Input: part model. Units: mm. Frame: model coordinates. A direction names the side the tool comes from. Round coordinates to 2 decimals unless told otherwise and drop trailing zeros. Order: outer loops, then holes, each group sorted by start corner. A loop starts at its lowest first (then second) coordinate and runs counter-clockwise, first axis right, second up.
Item 1: Mould query, pull axis Y, two halves, no side actions, for faces 1 (the cylindrical face through (8.4, 22.8, -1)), 2 (the flat face through (1, -26, -9)), 3 (the flat face through (10, 21.7, -1)), 4 (the flat face through (-15.5, 8, -6)). Classes: released by +Y, released by -Y, zero draft, split by the parting line, or undercut.
Item 2: First-contact query: pin 1 (2 mm diameter, centred on x = 2.5, z = -7.5, fed in from +Y); pin 2 (0.7 mm diameter, centred on x = -10, y = 22.5, fed in from +Z). Flat tips, straight axial feed; report the tip coordinate or a pass-through.
Item 3: Cut plane C-C on z = -10.5. Output: boundary loops of the cut face in (x, y), then the cut area to 3 significant figures.
Item 4: Reachability of faces 5 (the cylindrical face through (-8.65, 22.78, -0.99)), 6 (the flat face through (8, -25, -6)), 7 (the flat face through (6.5, 23, -7)), 8 (the cylindrical face through (-12.54, 24.65, -4.22)) from +Z, -Z, +X, -X, +Y, -Y: full face, straight path, thin tool, end or side. Return the list, or none.
Item 5: Cut plane A-A on z = -4.3. Output: boundary loops of the cut face in (x, y).
Item 6: Line query: L1, parallel to Z at x = 8.8, y = 22.8; L2, parallel to Z at x = 11.4, y = 22.8; L3, parallel to Y at x = -5, z = -10. Output: solid intervals per line, ascending.
Item 7: Cut plane D-D on y = 22.8. Give the number of separate pieces and of enclosed holes in the cut face, then the cut area to 3 significant figures.
Item 8: Cut plane B-B on x = 3. Output: boundary loops of the cut face in (y, z).
```python
from build123d import *

# Parameters (mm, degrees)
F0_W      = 31
F0_H      = 52
F1_DEPTH  = 12
F2_R      = 1.5
F3_DEPTH  = 25
F4_R      = 0.75
F5_DEPTH  = 2
F6_W      = 2
F6_H      = 0.2
F8_W      = 3
F8_H      = 16
F9_DEPTH  = 12.001
F10_W     = 13
F10_H     = 7
F11_DEPTH = 9.5
F12_R     = 1.85
F12_R_2   = 1.5
F13_DEPTH = 6
F14_R     = 1.85
F15_DEPTH = 6


with BuildPart() as f1:
    # F0 (on Top) → F1 (new body)
    with BuildSketch(Plane.XY):
        Rectangle(F0_W, F0_H)
    extrude(amount=-F1_DEPTH)

    # F2 (on Right) → F3 (cut, symmetric)
    with BuildSketch(Plane.YZ):
        with Locations((22.8, -4.3)):
            Circle(F2_R)
        with BuildLine():
            Line((-28.7, -6), (-23.7, -6))
            ThreePointArc((-23.7, -6), (-22, -4.3), (-23.7, -2.6))
            Line((-23.7, -2.6), (-28.7, -2.6))
            Line((-28.7, -2.6), (-28.7, -6))
        make_face()
    extrude(amount=F3_DEPTH, both=True, mode=Mode.SUBTRACT)

    # F4 (on face) → F5 (cut)
    with BuildSketch(Plane.XY):
        with BuildLine():
            Line((9.5, 21.7), (10.5, 21.7))
            ThreePointArc((10.5, 21.7), (11.6, 22.8), (10.5, 23.9))
            Line((10.5, 23.9), (9.5, 23.9))
            ThreePointArc((9.5, 23.9), (8.4, 22.8), (9.5, 21.7))
        make_face()
        with BuildLine():
            Line((-9.75, 23.9), (-10.25, 23.9))
            ThreePointArc((-10.25, 23.9), (-11.35, 22.8), (-10.25, 21.7))
            Line((-10.25, 21.7), (-9.75, 21.7))
            ThreePointArc((-9.75, 21.7), (-8.65, 22.8), (-9.75, 23.9))
        make_face()
        with Locations((-2.4, 22.8)):
            Circle(F4_R)
    extrude(amount=-F5_DEPTH, mode=Mode.SUBTRACT)

    # F6 (on face) → F7 (join, up to the next surface of F1)
    with BuildSketch(Plane.XZ.offset(26)):
        with Locations((0, -5.9)):
            Rectangle(F6_W, F6_H)
    extrude(until=Until.NEXT, dir=(0, 1, 0))

    # F8 (on face) → F9 (cut, through all)
    with BuildSketch(Plane.XY):
        with Locations((-14, -18)):
            Rectangle(F8_W, F8_H)
    extrude(amount=-F9_DEPTH, mode=Mode.SUBTRACT)

    # F10 (on face) → F11 (cut)
    with BuildSketch(Plane(origin=(0, 0, -12), x_dir=(1, 0, 0), z_dir=(0, 0, -1))):
        with Locations((0, -22.5)):
            Rectangle(F10_W, F10_H)
    extrude(amount=-F11_DEPTH, mode=Mode.SUBTRACT)

    # F12 (on face) → F13 (cut)
    with BuildSketch(Plane(origin=(-15.5, 0, 0), x_dir=(0, -1, 0), z_dir=(-1, 0, 0))):
        with Locations((-22.8, -4.3)):
            Circle(F12_R)
        with Locations((-22.8, -4.3)):
            Circle(F12_R_2, mode=Mode.SUBTRACT)
    extrude(amount=-F13_DEPTH, mode=Mode.SUBTRACT)

    # F14 (on face) → F15 (cut)
    with BuildSketch(Plane.YZ.offset(15.5)):
        with Locations((22.8, -4.3)):
            Circle(F14_R)
    extrude(amount=-F15_DEPTH, mode=Mode.SUBTRACT)


solid = f1.part
```
From the geometry:
1. face 1: undercut
1. face 2: released by -Y
1. face 3: undercut
1. face 4: zero draft
2. pin 1: stops at y = 19
2. pin 2: stops at z = -2
3. outline: (-15.5, -10) - (-12.5, -10) - (-12.5, -26) - (15.5, -26) - (15.5, 26) - (6.5, 26) - (6.5, 19) - (-6.5, 19) - (-6.5, 26) - (-15.5, 26) - close
3. area: 1,470 mm2
4. face 5: +Z
4. face 6: +X, -Y
4. face 7: -Z, +Y
4. face 8: -X
5. outline: (-15.5, -10) - (-12.5, -10) - (-12.5, -22) - (15.5, -22) - (15.5, 20.95) - (9.5, 20.95) - (9.5, 21.3) - (6.5, 21.3) - (6.5, 19) - (-6.5, 19) - (-6.5, 21.3) - (-9.5, 21.3) - (-9.5, 20.95) - (-15.5, 20.95) - close; (-15.5, 24.65) - (-9.5, 24.65) - (-9.5, 24.3) - (-6.5, 24.3) - (-6.5, 26) - (-15.5, 26) - close; (6.5, 24.3) - (9.5, 24.3) - (9.5, 24.65) - (15.5, 24.65) - (15.5, 26) - (6.5, 26) - close
6. L1: z = -12 to -5.8, -2.8 to -2
6. L2: z = -12 to -6.15, -2.45 to -2
6. L3: y = -26 to 19
7. separate pieces: 3
7. enclosed holes: 0
7. area: 171 mm2
8. outline: (-26, -12) - (19, -12) - (19, -2.5) - (26, -2.5) - (26, 0) - (-26, 0) - (-26, -2.6) - (-23.7, -2.6) arc R1.7 cw to (-23.7, -6) - (-26, -6) - close
